Design review of the part built by this model. Coordinates are the model's own, in mm. A direction names the side the tool comes from. Coordinates: 2 decimals unless noted, no trailing zeros. Write each loop counter-clockwise with the first axis right and the second up, starting at its lowest first coordinate (ties: lowest second). Pieces come first, ordered by that corner, then holes. Notation, with made-up numbers: M -25.5,21 L -14.5,21 A11 cw -14.5,31 Z; hole C 74,40.25 d3. An arc over 180 degrees is marked long. One line per question, with ' | ' between items.
from build123d import *

# Parameters (mm, degrees)
BASPROSKE_W         = 7
BASPROSKE_H         = 7.2
TOOTHCUT_DEPTH      = 13.356374873
TEETHCUTS_COUNT     = 16
TEETHCUTS_ANGLE     = 337.5
BORSKE_R            = 0.5
BORE_DEPTH          = 50.0000508
SKETCH_1_R          = 2.55
CUT_EXTRUDE_1_DEPTH = 13.234691538
EXTRUDE_1_DEPTH     = 3


with BuildPart() as part:
    # BasProSke → Base-Revolve (revolve)
    with BuildSketch(Plane(origin=(0, 0, 0), x_dir=(1, 0, 0), z_dir=(0, 1, 0)), mode=Mode.PRIVATE) as base_revolve_sk:
        with Locations((3.5, 3.6)):
            Rectangle(BASPROSKE_W, BASPROSKE_H)
    revolve(base_revolve_sk.sketch.rotate(Axis((-10, 0, 0), (1, 0, 0)), 180), axis=Axis((-10, 0, 0), (1, 0, 0)))

    # TooCutSke → ToothCut (cut, through all)
    with BuildSketch(Plane(origin=(0, 0, 0), x_dir=(0, 0, -1), z_dir=(1, 0, 0))):
        with BuildLine():
            ThreePointArc((0.418431057, 5.382761043), (0, 5.399), (-0.418431057, 5.382761043))
            ThreePointArc((-0.418431057, 5.382761043), (-0.663605074, 6.330572066), (-1.246629414, 7.117044349))
            ThreePointArc((-1.246629414, 7.117044349), (0, 7.2254), (1.246629414, 7.117044349))
            ThreePointArc((1.246629414, 7.117044349), (0.663605074, 6.330572066), (0.418431057, 5.382761043))
        make_face()
    toothcut = extrude(amount=TOOTHCUT_DEPTH, mode=Mode.SUBTRACT)

    # TeethCuts: ToothCut ×16 about axis
    teethcuts_axis = Axis((-10, 0, 0), (1, 0, 0))
    for i in range(1, TEETHCUTS_COUNT):
        add(toothcut.rotate(teethcuts_axis, i * TEETHCUTS_ANGLE / (TEETHCUTS_COUNT - 1)), mode=Mode.SUBTRACT)

    # BorSke → Bore (cut, symmetric)
    with BuildSketch(Plane(origin=(0, 0, 0), x_dir=(0, 0, -1), z_dir=(1, 0, 0))):
        with Locations(Location((0, 0, 0), (0, 0, 180))):
            Circle(BORSKE_R)
    extrude(amount=BORE_DEPTH, both=True, mode=Mode.SUBTRACT)

    # Sketch 1 → Cut-Extrude 1 (cut, through all)
    with BuildSketch(Plane(origin=(0, 0, 0), x_dir=(0, 0, -1), z_dir=(1, 0, 0))):
        Circle(SKETCH_1_R)
    extrude(amount=CUT_EXTRUDE_1_DEPTH, mode=Mode.SUBTRACT)

    # Sketch 2 → Extrude 1 (add)
    with BuildSketch(Plane.ZY.offset(-7)):
        with BuildLine():
            Line((-3.5, -1), (-2.345740821, -1))
            ThreePointArc((-2.345740821, -1), (-2.55, 0), (-2.345740821, 1))
            Line((-2.345740821, 1), (-3.5, 1))
            Line((-3.5, 1), (-3.5, -1))
        make_face()
        with BuildLine():
            Line((2.345740821, -1), (4.5, -1))
            Line((4.5, -1), (4.5, 1))
            Line((4.5, 1), (2.345740821, 1))
            ThreePointArc((2.345740821, 1), (2.498413406, 0.510323871), (2.55, 0))
            ThreePointArc((2.55, 0), (2.498413406, -0.510323871), (2.345740821, -1))
        make_face()
    extrude(amount=-EXTRUDE_1_DEPTH)


solid = part.part
1. To check wall thickness, follow line 1 along Z through (x, y) = (7.5, 0); line 2 along Z through (x, y) = (2, 3.75); line 3 along Y through (x, z) = (3.75, 5.5). State the ranges of each line that lie inside material, in increasing order. Write a range as [from, to].
Answer sheet:
line 1: [-3.5, -2.55], [2.55, 4.5] | line 2: [-6.05, -4.42], [-3.88, 3.88], [4.42, 6.05] | line 3: [-4.14, -2.94], [-1.77, -0.43], [0.43, 1.77], [2.94, 4.14]
2. Draft analysis for pull direction Y (two halves, no side actions). For faces 1 (the face through (3.45, 4.92, -4)), 2 (the face through (3.45, 5.57, 3.01)), 3 (the face through (8, 0, 4.5)), 4 (the face through (3.45, -5.59, 3.03)), state which applies: pulls with the +Y half, pulls with the -Y half, needs draft (parallel to the pull), parting line crosses it, or undercut.
Answer sheet:
face 1: undercut | face 2: pulls with the +Y half | face 3: needs draft | face 4: pulls with the -Y half
3. Take a section at A-A (x = 8.5). Write out the cut boundary in (y, z).
Answer sheet:
outline: M -1,-3.5 L 1,-3.5 L 1,-2.35 A2.55 cw -1,-2.35 Z; M -1,2.35 A2.55 cw 1,2.35 L 1,4.5 L -1,4.5 Z
4. Insertion check: pin 1 Ø1 at (x, z) = (8.5, -5) entering from +Y; pin 2 Ø2 at (x, z) = (1.5, -5) entering from +Y; pin 3 Ø0.6 at (x, z) = (9, 3.5) entering from +Y; pin 4 Ø0.6 at (x, z) = (9, 3.5) entering from -Y. Each pin has a flat end and moves straight along its axis. Give the tip position at first contact, or say it passes through.
Answer sheet:
pin 1: through | pin 2: y = 5.99 | pin 3: y = 1 | pin 4: y = -1
5. Take a section at B-B (z = 0). Write out the cut boundary in (x, y).
Answer sheet:
outline: M 0,-5.4 L 7,-5.4 L 7,-2.55 L 0,-2.55 Z; M 0,2.55 L 7,2.55 L 7,5.4 L 0,5.4 Z
6. Take a section at C-C (y = -4.5). Write out the cut boundary in (x, z), then the cut area to 3 significant figures.
Answer sheet:
outline: M 0,-3.8 L 7,-3.8 L 7,3.8 L 0,3.8 Z | area: 53.2 mm^2
7. Tool access review of faces 5 (the face through (3.45, -0.65, 6.3)), 6 (the face through (3.45, -6.3, -0.65)), 7 (the face through (3.451, -0.663, -6.328)), 8 (the face through (3.45, 1.81, 6.07)): name each direction out of +Z, -Z, +X, -X, +Y, -Y from which nothing blocks a thin tool from reaching the whole face with its end or side.
Answer sheet:
face 5: +Z, +X, -X | face 6: +X, -X, -Y | face 7: -Z, +X, -X | face 8: +X, -X
